from build123d import *

# Parameters (mm, degrees)
F1_DEPTH       = 70
F2_W           = 40
F2_H           = 20
F3_DEPTH       = 64
F6_DEPTH       = 20
F9_DEPTH       = 20
F11_DEPTH      = 70.001
F12_W          = 24
F12_H          = 53
F13_DEPTH      = 15.5455173281
F14_R          = 2
F15_DEPTH      = 15.5455173281
F16_DEPTH      = 10
F17_W          = 1.5
F17_H          = 9
F17_W_2        = 9
F17_H_2        = 1.5
F18_DEPTH      = 64
F19_SIZE       = 1.49999
F20_R          = 2.75
F21_DEPTH      = 41.501
F21_DEPTH_BACK = 78.501
F24_R          = 5.5
F25_DEPTH      = 36.001
F26_R          = 5.5
F27_DEPTH      = 36.001
F28_R          = 2.75
F29_DEPTH      = 4.001


# Not quite as in the source:
# - a fillet or chamfer is up to 0.001 mm smaller than in the source, because OpenCascade refuses the exact size


with BuildPart() as f1:
    # F0 (on Top) → F1 (new body)
    with BuildSketch(Plane.XY):
        Polygon((30, 51.9615242271), (0, 0), (120, 0), (90, 51.9615242271), align=None)
    extrude(amount=F1_DEPTH)

    # F2 (on face) → F3 (cut)
    with BuildSketch(Plane.XY.offset(70)):
        with Locations((60, 37.9615242271)):
            Rectangle(F2_W, F2_H)
    extrude(amount=-F3_DEPTH, mode=Mode.SUBTRACT)

    # F5 (on offset) → F6 (cut)
    with BuildSketch(Plane.XY.offset(4)):
        Polygon((19.6188021535, 25.9807621135), (4.6188021535, 0), (27.7128129211, 0), (36.9393102292, 15.9807621135), align=None)
        Polygon((100.3811978465, 25.9807621135), (83.0606897708, 15.9807621135), (92.2871870789, 0), (115.3811978465, 0), align=None)
    extrude(amount=F6_DEPTH, mode=Mode.SUBTRACT)

    # F8 (on offset) → F9 (cut)
    with BuildSketch(Plane.XY.offset(66)):
        Polygon((19.6188021535, 25.9807621135), (4.6188021535, 0), (27.7128129211, 0), (36.9393102292, 15.9807621135), align=None)
        Polygon((100.3811978465, 25.9807621135), (83.0606897708, 15.9807621135), (92.2871870789, 0), (115.3811978465, 0), align=None)
    extrude(amount=-F9_DEPTH, mode=Mode.SUBTRACT)

    # F10 (on face) → F11 (cut, through all)
    with BuildSketch(Plane.XY.offset(70)):
        Polygon((39.5, 12.416006899), (32.3316150746, 0), (87.6683849254, 0), (80.5, 12.416006899), align=None)
    extrude(amount=-F11_DEPTH, mode=Mode.SUBTRACT)

    # F12 (on face) → F13 (cut, through all)
    with BuildSketch(Plane.XZ.offset(-12.416006899)):
        with Locations((60, 35)):
            Rectangle(F12_W, F12_H)
    extrude(amount=-F13_DEPTH, mode=Mode.SUBTRACT)

    # F14 (on face) → F15 (cut, through all)
    with BuildSketch(Plane.XZ.offset(-12.416006899)):
        with Locations((44.5, 50.5)):
            Circle(F14_R)
        with Locations((44.5, 19.5)):
            Circle(F14_R)
        with Locations((75.5, 19.5)):
            Circle(F14_R)
        with Locations((75.5, 50.5)):
            Circle(F14_R)
    extrude(amount=-F15_DEPTH, mode=Mode.SUBTRACT)

    # F16 (cut): a face of the model
    f16_faces = [f1.faces().sort_by_distance(p)[0] for p in [
        (40.7547184906, 27.9615242271, 38),
    ]]
    extrude(f16_faces, amount=-F16_DEPTH, mode=Mode.SUBTRACT)

    # F17 (on face) → F18 (join, through all)
    with BuildSketch(Plane.XY.offset(70)):
        with Locations((40.75, 37.9615242271)):
            Rectangle(F17_W, F17_H)
        with Locations((50, 47.2115242271)):
            Rectangle(F17_W_2, F17_H_2)
        with Locations((79.25, 37.9615242271)):
            Rectangle(F17_W, F17_H)
        with Locations((70, 47.2115242271)):
            Rectangle(F17_W_2, F17_H_2)
    extrude(amount=-F18_DEPTH)

    # F19 (size 1.5 in the source; OpenCascade refuses exactly that, so slightly less here)
    f19_edges = [f1.edges().sort_by_distance(p)[0] for p in [
        (54.5, 46.461524, 38),
        (45.5, 46.461524, 38),
        (50, 46.461524, 70),
        (41.5, 37.961524, 70),
        (41.5, 33.461524, 38),
        (65.5, 46.461524, 38),
        (74.5, 46.461524, 38),
        (78.5, 33.461524, 38),
        (78.5, 42.461524, 38),
        (70, 46.461524, 70),
        (78.5, 37.961524, 70),
        (41.5, 42.461524, 38),
    ]]
    chamfer(f19_edges, length=F19_SIZE)

    # F20 (on face) → F21 (cut, two sides)
    with BuildSketch(Plane(origin=(78.5, 0, 0), x_dir=(0, -1, 0), z_dir=(-1, 0, 0))) as f21_sk:
        with Locations((-37.9615242271, 60)):
            Circle(F20_R)
        with Locations((-37.9615242271, 40)):
            Circle(F20_R)
        with Locations((-37.9615242271, 20)):
            Circle(F20_R)
    extrude(amount=-F21_DEPTH, mode=Mode.SUBTRACT)
    extrude(f21_sk.sketch, amount=F21_DEPTH_BACK, mode=Mode.SUBTRACT)

    # F24 (on offset) → F25 (cut, through all)
    with BuildSketch(Plane(origin=(84, 0, 0), x_dir=(0, -1, 0), z_dir=(-1, 0, 0))):
        with Locations((-37.9615242271, 60)):
            Circle(F24_R)
        with Locations((-37.9615242271, 40)):
            Circle(F24_R)
        with Locations((-37.9615242271, 20)):
            Circle(F24_R)
    extrude(amount=-F25_DEPTH, mode=Mode.SUBTRACT)

    # F26 (on offset) → F27 (cut, through all)
    with BuildSketch(Plane.YZ.offset(36)):
        with Locations((37.9615242271, 60)):
            Circle(F26_R)
        with Locations((37.9615242271, 40)):
            Circle(F26_R)
        with Locations((37.9615242271, 20)):
            Circle(F26_R)
    extrude(amount=-F27_DEPTH, mode=Mode.SUBTRACT)

    # F28 (on face) → F29 (cut, through all)
    with BuildSketch(Plane.XZ.offset(-47.9615242271)):
        with Locations((60, 60)):
            Circle(F28_R)
        with Locations((60, 40)):
            Circle(F28_R)
        with Locations((60, 20)):
            Circle(F28_R)
    extrude(amount=-F29_DEPTH, mode=Mode.SUBTRACT)


solid = f1.part
Geometry check sheet. Reference: the model listing, model coordinates, mm. A direction names the side the tool comes from. Give positions to 0.01 mm unless a question says otherwise; leave off trailing zeros. Order: outer loops, then holes, each group sorted by start corner. A loop starts at its lowest first (then second) coordinate and runs counter-clockwise, first axis right, second up. Notation, with made-up numbers: (24.5, 49.5) - (37.5, 49.5) arc R34 ccw to (37.5, 83.5) - close; hole circle Ø3 at (36, -14). An arc over 180 degrees is marked (long way). Use one line per item in the form item = value.
1) Sectioned sample at B-B (y = 29). Record the boundary of the cut face in (x, z).
Working result:
outline = (16.74, 0) - (103.26, 0) - (103.26, 70) - (80, 70) - (80, 6) - (40, 6) - (40, 70) - (16.74, 70) - close
2) Sectioned sample at A-A (x = 60). Record the boundary of the cut face in (y, z).
Working result:
outline = (12.42, 0) - (51.96, 0) - (51.96, 17.25) - (47.96, 17.25) - (47.96, 6) - (17.96, 6) - (17.96, 8.5) - (12.42, 8.5) - close; (12.42, 61.5) - (17.96, 61.5) - (17.96, 70) - (12.42, 70) - close; (47.96, 22.75) - (51.96, 22.75) - (51.96, 37.25) - (47.96, 37.25) - close; (47.96, 42.75) - (51.96, 42.75) - (51.96, 57.25) - (47.96, 57.25) - close; (47.96, 62.75) - (51.96, 62.75) - (51.96, 70) - (47.96, 70) - close
3) Access from +Z, -Z, +X, -X, +Y, -Y to the whole of each face (thin tool, end or side, straight path). Record for faces 4 (the face through (57.973, 49.934, 61.859)), 5 (the face through (44.24, 15.15, 21.483)), 6 (the face through (90.591, 32.881, 17.893)), 7 (the face through (32.261, 7.879, 56.14)).
Working result:
face_4 = +Y
face_5 = -Y
face_6 = +X
face_7 = none
4) Draft check along X on faces 1 (the face through (91.84, 21.05, 13.86)), 2 (the face through (105.21, 25.62, 34.51)), 3 (the face through (38.788, 36.483, 62.319)). Enter one of: released by +X, released by -X, zero draft, split by the parting line, or undercut.
Working result:
face_1 = undercut
face_2 = released by +X
face_3 = zero draft
5) Sectioned sample at D-D (z = 40). Count the separate pieces of the cut face and the enclosed holes in it, and give its area (3 significant figures).
Working result:
separate_pieces = 4
enclosed_holes = 0
area = 2,400 mm^2
6) Sectioned sample at C-C (x = 99). Record the boundary of the cut face in (y, z), and give its area (3 significant figures).
Working result:
outline = (0, 0) - (36.37, 0) - (36.37, 14.73) arc R5.5 cw to (36.37, 25.27) - (36.37, 34.73) arc R5.5 cw to (36.37, 45.27) - (36.37, 54.73) arc R5.5 cw to (36.37, 65.27) - (36.37, 70) - (0, 70) - (0, 66) - (25.18, 66) - (25.18, 46) - (0, 46) - (0, 24) - (25.18, 24) - (25.18, 4) - (0, 4) - close
area = 1,450 mm^2
7) Material ranges on probe 1 along Z at (x, y) = (17.5, 7); probe 2 along Z at (x, y) = (60, 51.05); probe 3 along Z at (x, y) = (44.5, 14.85), recorded low to high. Write a range as from..to.
Working result:
probe_1 = 0..4, 24..46, 66..70
probe_2 = 0..17.25, 22.75..37.25, 42.75..57.25, 62.75..70
probe_3 = 0..17.5, 21.5..48.5, 52.5..70
8) Depth check by flat-ended pin: pin 1 Ø4 at (x, y) = (53, 39.5) entering from -Z; pin 2 Ø6 at (x, z) = (43, 37.5) entering from -Y; pin 3 Ø1.8 at (y, z) = (38.5, 49.5) entering from -X; pin 4 Ø3.5 at (y, z) = (37.96, 40) entering from -X. Enter the tip coordinate at first touch or a pass-through.
Working result:
pin_1 = 0
pin_2 = 12.42
pin_3 = 21.71
pin_4 = through
